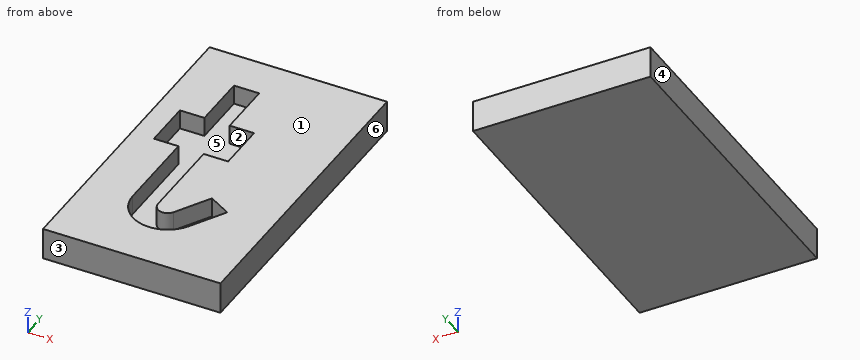
from build123d import *

# Parameters (mm, degrees)
F0_W     = 72.546231
F0_H     = 128.329664
F1_DEPTH = 13
F3_DEPTH = 8


# Not quite as in the source:
# - ends of sketch curves that miss each other by under 0.0002 mm in the source are joined


with BuildPart() as f1:
    # F0 (on Top) → F1 (new body)
    with BuildSketch(Plane.XY):
        with Locations((5e-07, 0)):
            Rectangle(F0_W, F0_H)
    extrude(amount=F1_DEPTH)

    # F2 (on face) → F3 (cut)
    with BuildSketch(Plane.XY.offset(13)):
        with BuildLine():
            Line((-6.941915, 24.355961), (-6.941915, 47.164832))
            Line((-6.941915, 47.164832), (-17.273115, 47.164832))
            Line((-17.273115, 47.164832), (-17.273115, 24.355961))
            Line((-17.273115, 24.355961), (-27.273115, 24.355961))
            Line((-27.273115, 24.355961), (-27.273115, 4.355961))
            Line((-27.273115, 4.355961), (-17.273115, 4.355961))
            Line((-17.273115, 4.355961), (-17.2731146267, -30.8336322155))
            Line((-17.2731146267, -30.8336322155), (-17.2731146267, -30.8377282155))
            Line((-17.2731146267, -30.8377282155), (-17.2731139504, -30.8380352155))
            ThreePointArc((-17.2731139504, -30.8380352155), (-6.6489757762, -44.6770778186), (9.4692682, -37.9992321155))
            Line((9.4692682, -37.9992321155), (17.6391412, -23.8485971155))
            Line((17.6391412, -23.8485971155), (8.69206, -18.682997))
            Line((8.69206, -18.682997), (0.522187, -32.833632))
            ThreePointArc((0.522187, -32.833632), (-3.9764490293, -34.6975341769), (-6.9419144165, -30.8351679998))
            Line((-6.9419144165, -30.8351679998), (-6.94191496, -30.8348611666))
            Line((-6.94191496, -30.8348611666), (-6.94191496, -30.8336322155))
            Line((-6.94191496, -30.8336322155), (-6.94191496, 4.355961))
            Line((-6.94191496, 4.355961), (3.058085, 4.355961))
            Line((3.058085, 4.355961), (3.05808504, 24.355961))
            Line((3.05808504, 24.355961), (-6.941915, 24.355961))
        make_face()
    extrude(amount=-F3_DEPTH, mode=Mode.SUBTRACT)


solid = f1.part
The listing builds one solid part. Answer for the finished solid, in the listing's coordinates (mm). Face numbers are marked on the shaded views. A direction names the side the tool comes from. Coordinates: 2 decimals unless noted, no trailing zeros. Write each loop counter-clockwise with the first axis right and the second up, starting at its lowest first coordinate (ties: lowest second). Pieces come first, ordered by that corner, then holes. Notation, with made-up numbers: M 41,-36.5 L 56,-36.5 A20 cw 56,-7.5 Z; hole C -15,-17 d6. An arc over 180 degrees is marked long. Use one line per item in the form item = value.
Item 1: Find the intervals of material crossed by probe 1 along X at (y, z) = (16, 11); probe 2 along Y at (x, z) = (-18.5, 7); probe 3 along X at (y, z) = (-14, 8), in increasing order.
Model answer:
probe_1 = -36.27 to -27.27, 3.06 to 36.27
probe_2 = -64.16 to 4.36, 24.36 to 64.16
probe_3 = -36.27 to -17.27, -6.94 to 36.27
Item 2: The mould has two halves that part along X. Classify the marked faces 3, 4, 5 and 6: released by +X, released by -X, zero draft, split by the parting line, or undercut.
Model answer:
face_3 = zero draft
face_4 = released by -X
face_5 = undercut
face_6 = released by +X
Item 3: Find section C-C, the plane y = -28.5. Give the vertices of the cut face in (x, z), plus the area to 3 significant figures.
Model answer:
outline = M -36.27,0 L 36.27,0 L 36.27,13 L 14.95,13 L 14.95,5 L 3.02,5 L 3.02,13 L -6.94,13 L -6.94,5 L -17.27,5 L -17.27,13 L -36.27,13 Z
area = 765 mm2
Item 4: Find section D-D, the plane x = 11. Give the vertices of the cut face in (y, z), plus the area to 3 significant figures.
Model answer:
outline = M -64.16,0 L 64.16,0 L 64.16,13 L -20.02,13 L -20.02,5 L -35.35,5 L -35.35,13 L -64.16,13 Z
area = 1,550 mm2
Item 5: For the marked faces 1 and 2, determine the directions among +Z, -Z, +X, -X, +Y, -Y from which every point of the face is accessible in a straight line to the end or side of a thin tool.
Model answer:
face_1 = +Z, +X, -X, +Y, -Y
face_2 = +Z
Item 6: Find section B-B, the plane x = -23. Give the vertices of the cut face in (y, z).
Model answer:
outline = M -64.16,0 L 64.16,0 L 64.16,13 L 24.36,13 L 24.36,5 L 4.36,5 L 4.36,13 L -64.16,13 Z
